Autodesk Inventor part; units mm, degrees
ref_plane "XZ Plane" through (0, 0, 0) normal (0, 1, 0) x (-1, 0, 0)
ref_plane "XY Plane" through (0, 0, 0) normal (0, 0, 1) x (1, 0, 0)
sketch "Sketch1" plane through (0, 0, 0) normal (0, 0, 1) x (1, 0, 0)
  circle A0 centre (0, 35.5533) radius 2.1
  circle A1 centre (11, 25.3552) radius 2.1
  circle A2 centre (-11, 25.3552) radius 2.1
  circle A3 centre (6.25, -60.9016) radius 2.1
  circle A4 centre (-33.6286, -15.6738) radius 2.1
  circle A5 centre (-5.75, -60.9016) radius 2.1
  circle A6 centre (34.1286, -15.6738) radius 2.1
  circle A7 centre (-24.1373, -40.1344) radius 6.75
  circle A8 centre (24.6373, -40.1344) radius 6.75
  circle A9 centre (10.7484, -21.5639) radius 2.1
  circle A10 centre (-10.2484, -21.5639) radius 2.1
  line L0 (-59, -41.44) -> (-59, -14.3421)
  line L1 (-59, -41.44) -> (-53, -41.44)
  line L2 (-53, -41.44) -> (-53, -91.44)
  line L3 (-53, -91.44) -> (53, -91.44)
  line L4 (53, -91.44) -> (53, -41.44)
  line L5 (53, -41.44) -> (59, -41.44)
  line L6 (59, -14.3421) -> (59, -41.44)
  line L7 (59, -14.3421) -> (54, -14.3421)
  line L8 (54, -14.3421) -> (54, 35.0192)
  line L9 (54, 35.0192) -> (59, 35.0192)
  line L10 (59, 80.19) -> (59, 35.0192)
  line L11 (59, 80.19) -> (46.35, 80.19)
  line L12 (46.35, 80.19) -> (46.35, 63.44)
  line L13 (46.35, 63.44) -> (-46.35, 63.44)
  line L14 (-46.35, 63.44) -> (-46.35, 80.19)
  line L15 (-46.35, 80.19) -> (-59, 80.19)
  line L16 (-59, 35.0192) -> (-59, 80.19)
  line L17 (-59, 35.0192) -> (-54, 35.0192)
  line L18 (-54, 35.0192) -> (-54, -14.3421)
  line L19 (-54, -14.3421) -> (-59, -14.3421)
  circle A11 centre (0, 35.5533) radius 6.1 construction
  line L20 (34.1312, 49.9126) -> (34.1312, 18.1374) construction
  line L21 (-34.1313, 18.1374) -> (-34.1313, 49.9126) construction
  line L22 (34.1312, 43.6533) -> (-34.1313, 43.6533)
  line L23 (-34.1313, 43.6533) -> (-34.1312, 29.7711)
  line L24 (-30.0745, -3.9522) -> (30.0745, -3.9522)
  line L25 (34.1312, 29.7711) -> (34.1312, 43.6533)
  line L26 (-30, -3.9121) -> (30, -3.9121) construction
  line L27 (30, -3.9121) -> (30, 36.0879) construction
  line L28 (30, 36.0879) -> (-30, 36.0879) construction
  line L29 (-30, 36.0879) -> (-30, -3.9121) construction
  line L30 (-30, -3.9121) -> (30, 36.0879) construction
  line L31 (30, -3.9121) -> (-30, 36.0879) construction
  line L32 (-34.1312, 29.7711) -> (-30.0745, -3.9522)
  line L33 (0, 16.0879) -> (0, 8.3045) construction
  line L34 (34.1312, 29.7711) -> (30.0745, -3.9522)
  line L35 (26.5268, 0.0478) -> (-26.5268, 0.0478)
  line L36 (-26.5268, 0.0478) -> (-30.1312, 30.0109)
  line L37 (-30.1312, 30.0109) -> (-30.1312, 39.6533)
  line L38 (-30.1312, 39.6533) -> (30.1312, 39.6533)
  line L39 (30.1312, 39.6533) -> (30.1312, 30.0109)
  line L40 (30.1312, 30.0109) -> (26.5268, 0.0478)
  line L41 (-28.8342, 19.2288) -> (28.8342, 19.2288)
  line L42 (-27.0103, 4.0668) -> (-22.9193, 0.0478)
  line L43 (27.0103, 4.0668) -> (22.9193, 0.0478)
  point P0 (0, 0)
  point P1 (30.0601, -3.9522)
  point P2 (34.1312, 29.891)
  point P3 (22.9193, 0.0478)
  dimension "d0" = 4
  dimension "d3" = 60
  dimension "d4" = 40
  dimension "d5" = 4
extrude "Extrusion1" add sketch "Sketch1" along normal blind 4 contours L25 L34 L24 L32 L23 L22 | L35 L43 L40 | L35 L36 L42 | L41 L36 L37 L38 L39 L40
sketch "Sketch2" plane through (0, 0, 4) normal (0, 0, 1) x (1, 0, 0)
  line L0 (-30, 36.0478) -> (30, 36.0478)
  line L1 (30, 36.0478) -> (30, -3.9522)
  line L2 (30, -3.9522) -> (-30, -3.9522)
  line L3 (-30, -3.9522) -> (-30, 36.0478)
  line L4 (-30, 36.0478) -> (30, -3.9522) construction
  line L5 (30, 36.0478) -> (-30, -3.9522) construction
  line L6 (-30.0745, -3.9522) -> (30.0745, -3.9522) construction
  circle A0 centre (27.15, -1.1022) radius 1 construction
  circle A1 centre (27.15, -1.1022) radius 1.2
  circle A2 centre (27.15, -1.1022) radius 2.85
  line L7 (30, 16.0478) -> (-30, 16.0478) construction
  line L8 (0, 36.0478) -> (0, -3.9522) construction
  circle A3 centre (27.15, 33.1978) radius 1.2
  circle A4 centre (27.15, 33.1978) radius 2.85
  circle A5 centre (-27.15, -1.1022) radius 1.2
  circle A6 centre (-27.15, -1.1022) radius 2.85
  circle A7 centre (-27.15, 33.1978) radius 1.2
  circle A8 centre (-27.15, 33.1978) radius 2.85
  point P0 (0, 0)
  point P1 (0, 16.0478)
  dimension "d6" = 60
  dimension "d7" = 40
  dimension "d8" = 2
  dimension "d9" = 2.85
  dimension "d10" = 2.85
  dimension "d11" = 0.2
extrude "Extrusion2" add sketch "Sketch2" along normal blind 5 contours A8 | A4 | A6 | A2
sketch "Sketch3" plane through (-34.1312, 29.7711, 0) normal (-1, 0, 0) x (0, 0, 1)
  line L0 (4, 13.8821) -> (4, 0)
  line L1 (4, 13.8821) -> (24, 13.8821)
  line L2 (24, 13.8821) -> (24, 8.5067)
  line L3 (24, 8.5067) -> (4, 8.5067)
  line L4 (4, 8.5067) -> (4, 13.8821)
  line L5 (24, 13.8821) -> (26.8284, 16.7106)
  line L6 (24, 13.8821) -> (28, 13.8821) construction
  line L7 (26.8284, 16.7106) -> (26.8284, 8.5067)
  line L8 (26.8284, 8.5067) -> (24, 8.5067)
  point P0 (0, -29.7711)
  point P1 (4, 8.5067)
  dimension "d14" = 20
  dimension "d15" = 4
  dimension "d16" = 45
extrude "Extrusion3" add sketch "Sketch3" against normal blind 20
chamfer "Chamfer1" distance 3.175 angle 45 1 edges at (-24.1313, 38.2779, 26.8284)
chamfer "Chamfer2" distance 2 angle 45 6 edges at (-32.1029, 12.9095, 0) (0, -3.9522, 0) (32.1029, 12.9095, 0) (34.1312, 36.7122, 0) (0, 43.6533, 0) (-34.1313, 36.7122, 0)
fillet "Fillet1" radius 3.175 2 edges at (28.8342, 19.2288, 2) (-28.8342, 19.2288, 2)
mirror "Mirror1" about plane through (0, 0, 0) normal (1, 0, 0) of "Extrusion3", "Chamfer1"
equation "\"d10\" = d9"
properties part number "Esp32_Holder"
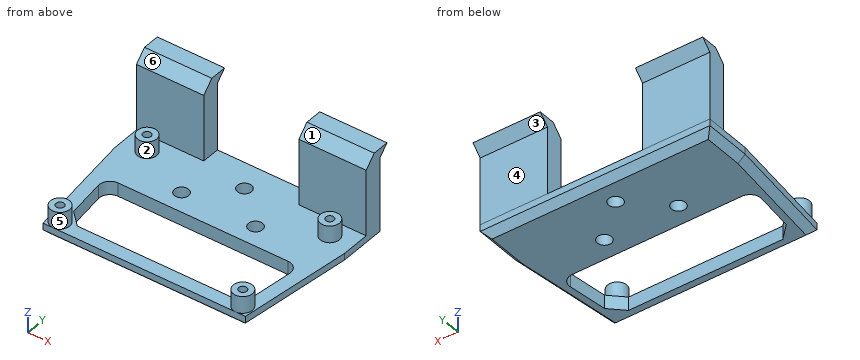
Geometry check sheet. Reference: the model listing, model coordinates, mm. Face numbers are marked on the shaded views. A direction names the side the tool comes from. Coordinates: 2 decimals unless noted, no trailing zeros. Order: outer loops, then holes, each group sorted by start corner. A loop starts at its lowest first (then second) coordinate and runs counter-clockwise, first axis right, second up. Notation, with made-up numbers: M 16.25,-34 L 28.25,-34 A8 ccw 28.25,-21 Z; hole C 65,81.25 d3. An arc over 180 degrees is marked long. One line per question, with ' | ' between items. Start each with the question number.
Item 1: Gauge pin test, flat ends, axial feed: pin 1 (1.4 mm diameter, centred on x = 27.15, y = -1.1, fed in from -Z); pin 2 (4.5 mm diameter, centred on x = 26.5, y = -1.5, fed in from +Z); pin 3 (4 mm diameter, centred on x = -11, y = 25.36, fed in from +Z); pin 4 (4 mm diameter, centred on x = 6, y = 17.5, fed in from +Z). Record the tip position at first contact, or that the pin passes through.
Item 2: Cross-section at A-A on z = 22. Enter the section's corners in (x, y), then the cut area to 3 significant figures.
Item 3: Draft check along Y on the marked faces 1, 2 and 3. Enter one of: pulls with the +Y half, pulls with the -Y half, needs draft (parallel to the pull), parting line crosses it, or undercut.
Item 4: Cross-section at D-D on x = 8. Enter the section's corners in (y, z), then the cut area to 3 significant figures.
Item 5: Cross-section at C-C on y = 13. Enter the section's corners in (x, z), then the cut area to 3 significant figures.
Item 6: Material ranges on L1, parallel to Y at x = 27.15, z = 6.9; L2, parallel to X at y = 40, z = 13.75; L3, parallel to Y at x = 0, z = 1.5, recorded low to high. Write a range as [from, to].
Item 7: Set-up check for the marked faces 4, 5 and 6: record each of +Z, -Z, +X, -X, +Y, -Y from which the full face is reachable in a straight line by a thin tool's end or side.
Findings:
1) pin 1: stops at z = 0 | pin 2: stops at z = 9 | pin 3: passes through | pin 4: stops at z = 4
2) outline: M -34.13,38.28 L -14.13,38.28 L -14.13,43.65 L -34.13,43.65 Z; M 14.13,38.28 L 34.13,38.28 L 34.13,43.65 L 14.13,43.65 Z | area: 215 mm²
3) face 1: pulls with the -Y half | face 2: undercut | face 3: pulls with the +Y half
4) outline: M -3.95,2 L -1.95,0 L 0.05,0 L 0.05,4 L -3.95,4 Z; M 19.23,0 L 41.65,0 L 43.65,2 L 43.65,4 L 19.23,4 Z | area: 110 mm²
5) outline: M -32.11,2 L -30.1,0 L -28.08,0 L -28.08,4 L -32.11,4 Z; M 28.08,0 L 30.1,0 L 32.11,2 L 32.11,4 L 28.08,4 Z | area: 28.2 mm²
6) L1: y = [-3.95, -2.3], [0.1, 1.75], [30.35, 32], [34.4, 36.05], [38.28, 43.65] | L2: x = [-34.13, -14.13], [14.13, 34.13] | L3: y = [-3.45, 0.05], [19.23, 33.45], [37.65, 43.15]
7) face 4: -Z, +X, -X, +Y | face 5: +Z | face 6: +Z, +X, -X, -Y
